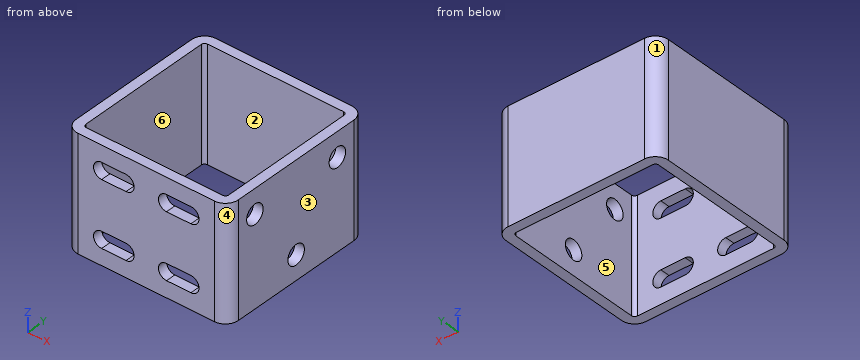
from build123d import *

# Parameters (mm, degrees)
EXTRUDE_1_DEPTH             = 70
CUT_EXTRUDE_1_REACH         = 102
SKETCH_2_R                  = 6
CUT_EXTRUDE_2_DEPTH         = 6
PATTERN_LINEAR_1_COUNT      = 2
PATTERN_LINEAR_1_PITCH      = 40
PATTERN_LINEAR_1_COUNT_DIR2 = 2
PATTERN_LINEAR_1_PITCH_DIR2 = 40


with BuildPart() as part:
    # 草图1 → 凸台-拉伸1 (new body)
    with BuildSketch(Plane.XY):
        with BuildLine():
            Line((8, 0), (92, 0))
            ThreePointArc((92, 0), (97.656854249, 2.343145751), (100, 8))
            Line((100, 8), (100, 92))
            ThreePointArc((100, 92), (97.656854249, 97.656854249), (92, 100))
            Line((92, 100), (8, 100))
            ThreePointArc((8, 100), (2.343145751, 97.656854249), (0, 92))
            Line((0, 92), (0, 8))
            ThreePointArc((0, 8), (2.343145751, 2.343145751), (8, 0))
        make_face()
        with BuildLine():
            Line((8, 94), (92, 94))
            ThreePointArc((92, 94), (93.414213562, 93.414213562), (94, 92))
            Line((94, 92), (94, 8))
            ThreePointArc((94, 8), (93.414213562, 6.585786438), (92, 6))
            Line((92, 6), (8, 6))
            ThreePointArc((8, 6), (6.585786438, 6.585786438), (6, 8))
            Line((6, 8), (6, 92))
            ThreePointArc((6, 92), (6.585786438, 93.414213562), (8, 94))
        make_face(mode=Mode.SUBTRACT)
    extrude(amount=EXTRUDE_1_DEPTH)

    # 草图2 → 切除-拉伸1 (cut, up to next)
    with BuildSketch(Plane(origin=(100, 0, 0), x_dir=(0, 0, -1), z_dir=(1, 0, 0)), mode=Mode.PRIVATE) as cut_extrude_1_sk1:
        with Locations((-55, 80)):
            Circle(SKETCH_2_R)
    cut_extrude_1_tool1 = extrude(cut_extrude_1_sk1.sketch, amount=-CUT_EXTRUDE_1_REACH, mode=Mode.PRIVATE) & part.part
    add(cut_extrude_1_tool1.solids().sort_by_distance((100, 80, 55))[0], mode=Mode.SUBTRACT)
    # 草图2 → 切除-拉伸1 (cut, up to next)
    with BuildSketch(Plane(origin=(100, 0, 0), x_dir=(0, 0, -1), z_dir=(1, 0, 0)), mode=Mode.PRIVATE) as cut_extrude_1_sk2:
        with Locations((-55, 20)):
            Circle(SKETCH_2_R)
    cut_extrude_1_tool2 = extrude(cut_extrude_1_sk2.sketch, amount=-CUT_EXTRUDE_1_REACH, mode=Mode.PRIVATE) & part.part
    add(cut_extrude_1_tool2.solids().sort_by_distance((100, 20, 55))[0], mode=Mode.SUBTRACT)
    # 草图2 → 切除-拉伸1 (cut, up to next)
    with BuildSketch(Plane(origin=(100, 0, 0), x_dir=(0, 0, -1), z_dir=(1, 0, 0)), mode=Mode.PRIVATE) as cut_extrude_1_sk3:
        with Locations((-15, 50)):
            Circle(SKETCH_2_R)
    cut_extrude_1_tool3 = extrude(cut_extrude_1_sk3.sketch, amount=-CUT_EXTRUDE_1_REACH, mode=Mode.PRIVATE) & part.part
    add(cut_extrude_1_tool3.solids().sort_by_distance((100, 50, 15))[0], mode=Mode.SUBTRACT)

    # 草图3 → 切除-拉伸2 (cut)
    with BuildSketch(Plane.XZ):
        with BuildLine():
            Line((77.5, 60), (62.5, 60))
            ThreePointArc((62.5, 60), (57.5, 55), (62.5, 50))
            Line((62.5, 50), (77.5, 50))
            ThreePointArc((77.5, 50), (82.5, 55), (77.5, 60))
        make_face()
    cut_extrude_2 = extrude(amount=-CUT_EXTRUDE_2_DEPTH, mode=Mode.SUBTRACT)

    # 阵列(线性)1: Cut-Extrude 2 2 × 2
    with Locations(*[(-j * PATTERN_LINEAR_1_PITCH_DIR2, 0, -i * PATTERN_LINEAR_1_PITCH) for i in range(PATTERN_LINEAR_1_COUNT) for j in range(PATTERN_LINEAR_1_COUNT_DIR2) if (i, j) != (0, 0)]):
        add(cut_extrude_2, mode=Mode.SUBTRACT)


solid = part.part
Verification items for the finished model (mm, model axes). Face numbers are marked on the shaded views. A direction names the side the tool comes from. Coordinates: 2 decimals unless noted, no trailing zeros. Write each loop counter-clockwise with the first axis right and the second up, starting at its lowest first coordinate (ties: lowest second). Pieces come first, ordered by that corner, then holes. Notation, with made-up numbers: M 51.25,72 L 89.25,72 A11 ccw 89.25,80 Z; hole C 13.25,88 d2. An arc over 180 degrees is marked long. Use a Markdown table: item, result.
Q1. Go/stop test with flat-tipped pins: P1, Ø11, axis at y = 80, z = 55, coming from the +X side; P2, Ø5, axis at x = 32, y = 3, coming from the -Z side; P3, Ø10, axis at x = 12.5, y = 45.5, coming from the +Z side. Record where each tip stops, or that it passes through.
Reply:
| item | result |
|---|---|
| P1 | stops at x = 6 |
| P2 | stops at z = 0 |
| P3 | passes through |
Q2. Sectioned sample at B-B, the plane y = 80. Record the boundary of the cut face in (x, z), plus the area to 3 significant figures.
Reply:
| item | result |
|---|---|
| outline | M 0,0 L 6,0 L 6,70 L 0,70 Z; M 94,0 L 100,0 L 100,49 L 94,49 Z; M 94,61 L 100,61 L 100,70 L 94,70 Z |
| area | 768 mm² |
Q3. Sectioned sample at A-A, the plane z = 55. Count the separate pieces of the cut face and the enclosed holes in it, plus the area to 3 significant figures.
Reply:
| item | result |
|---|---|
| separate pieces | 4 |
| enclosed holes | 0 |
| area | 1,760 mm² |
Q4. Sectioned sample at C-C, the plane x = 9.5. Record the boundary of the cut face in (y, z), plus the area to 3 significant figures.
Reply:
| item | result |
|---|---|
| outline | M 0,0 L 6,0 L 6,70 L 0,70 Z; M 94,0 L 100,0 L 100,70 L 94,70 Z |
| area | 840 mm² |
Q5. Draft check along Y on the marked faces 3, 4, 5 and 6. Enter one of: +Y half, -Y half, draft (parallel to the pull), parting line (faces both ways), or undercut.
Reply:
| item | result |
|---|---|
| face 3 | draft |
| face 4 | -Y half |
| face 5 | undercut |
| face 6 | undercut |
Q6. Set-up check for the marked faces 1 and 2: record each of +Z, -Z, +X, -X, +Y, -Y from which the full face is reachable in a straight line by a thin tool's end or side.
Reply:
| item | result |
|---|---|
| face 1 | +Z, -Z, -X, +Y |
| face 2 | +Z, -Z |
Q7. Thickness scan on line 1 (Y direction, x = 83, z = 32); line 2 (Y direction, x = 97, z = 55) (3 decimals). Record the ranges inside material, lowest first.
Reply:
| item | result |
|---|---|
| line 1 | y = 0 to 6, 94 to 100 |
| line 2 | y = 1.755 to 14, 26 to 74, 86 to 98.245 |
